Geometry check sheet. Reference: the model listing, model coordinates, mm. Give positions to 0.01 mm unless a question says otherwise; leave off trailing zeros. Order: outer loops, then holes, each group sorted by start corner. A loop starts at its lowest first (then second) coordinate and runs counter-clockwise, first axis right, second up.
from build123d import *

# Parameters (mm, degrees)
SKETCH1_W           = 96
SKETCH1_H           = 2
BOSS_EXTRUDE1_DEPTH = 98
SKETCH2_W           = 10
SKETCH2_H           = 2
BOSS_EXTRUDE2_DEPTH = 2
SKETCH3_W           = 10
SKETCH3_H           = 2
BOSS_EXTRUDE3_DEPTH = 2
SKETCH4_W           = 10
SKETCH4_H           = 2
BOSS_EXTRUDE4_DEPTH = 2


with BuildPart() as part:
    # Sketch1 → Boss-Extrude1 (new body)
    with BuildSketch(Plane.XY):
        with Locations((0, -49)):
            Rectangle(SKETCH1_W, SKETCH1_H)
    extrude(amount=BOSS_EXTRUDE1_DEPTH)

    # Sketch2 → Boss-Extrude2 (add)
    with BuildSketch(Plane.ZY.offset(48)):
        with Locations((73, -49)):
            Rectangle(SKETCH2_W, SKETCH2_H)
    boss_extrude2 = extrude(amount=BOSS_EXTRUDE2_DEPTH)

    # Mirror1: Boss-Extrude2 across plane
    add(boss_extrude2.mirror(Plane.XY.offset(50)))

    # Sketch3 → Boss-Extrude3 (add)
    with BuildSketch(Plane(origin=(48, 0, 0), x_dir=(0, 0, -1), z_dir=(1, 0, 0))):
        with Locations((-73, -49)):
            Rectangle(SKETCH3_W, SKETCH3_H)
    boss_extrude3 = extrude(amount=BOSS_EXTRUDE3_DEPTH)

    # Mirror2: Boss-Extrude3 across plane
    add(boss_extrude3.mirror(Plane.XY.offset(50)))

    # Sketch4 → Boss-Extrude4 (add)
    with BuildSketch(Plane(origin=(0, 0, 0), x_dir=(-1, 0, 0), z_dir=(0, 0, -1))):
        with Locations((23, -49)):
            Rectangle(SKETCH4_W, SKETCH4_H)
    boss_extrude4 = extrude(amount=BOSS_EXTRUDE4_DEPTH)

    # Mirror3: Boss-Extrude4 across plane
    add(boss_extrude4.mirror(Plane(origin=(0, 0, 0), x_dir=(0, 0, 1), z_dir=(1, 0, 0))))


solid = part.part
Item 1: Sectioned sample at C-C (z = 51.5). Enter the section's corners in (x, y), and give its area (3 significant figures).
Reported:
outline: (-48, -50) - (48, -50) - (48, -48) - (-48, -48) - close
area: 192 mm2
Item 2: Scan lines: L1, parallel to X at y = -49.3, z = 67; L2, parallel to Z at x = -7, y = -48.25. Record each from-to range of solid material in increasing order.
Reported:
L1: x = -48 to 48
L2: z = 0 to 98
Item 3: Sectioned sample at A-A (y = -48.95). Enter the section's corners in (x, z).
Reported:
outline: (-50, 22) - (-48, 22) - (-48, 0) - (-28, 0) - (-28, -2) - (-18, -2) - (-18, 0) - (18, 0) - (18, -2) - (28, -2) - (28, 0) - (48, 0) - (48, 22) - (50, 22) - (50, 32) - (48, 32) - (48, 68) - (50, 68) - (50, 78) - (48, 78) - (48, 98) - (-48, 98) - (-48, 78) - (-50, 78) - (-50, 68) - (-48, 68) - (-48, 32) - (-50, 32) - close
Item 4: Sectioned sample at B-B (x = -14.5). Enter the section's corners in (y, z), and give its area (3 significant figures).
Reported:
outline: (-50, 0) - (-48, 0) - (-48, 98) - (-50, 98) - close
area: 196 mm2
Item 5: Gauge pin test, flat ends, axial feed: pin 1 (1 mm diameter, centred on y = -49.5, z = 55, fed in from +X); pin 2 (1 mm diameter, centred on x = 49.5, y = -49.5, fed in from -Z); pin 3 (0.6 mm diameter, centred on x = -49, y = -49, fed in from +Z). Record the tip position at first contact, or that the pin passes through.
Reported:
pin 1: stops at x = 48
pin 2: stops at z = 22
pin 3: stops at z = 78
